The model under review builds one solid part; all positions refer to its coordinate system, in mm. Coordinates: 2 decimals unless noted, no trailing zeros. Write each loop counter-clockwise with the first axis right and the second up, starting at its lowest first coordinate (ties: lowest second). Pieces come first, ordered by that corner, then holes. Notation, with made-up numbers: M 76.5,-32 L 118.5,-32 A21 cw 118.5,-14 Z; hole C -36.5,-17 d3. An arc over 180 degrees is marked long. Answer as a JSON object with one key per item and string values.
Autodesk Inventor part; units mm, degrees
ref_plane "YZ Plane" through (0, 0, 0) normal (1, 0, 0) x (0, 1, 0)
ref_plane "XZ Plane" through (0, 0, 0) normal (0, 1, 0) x (-1, 0, 0)
ref_plane "XY Plane" through (0, 0, 0) normal (0, 0, 1) x (1, 0, 0)
sketch "Sketch1" plane through (0, 0, 0) normal (1, 0, 0) x (0, 1, 0)
  line L0 (0, 0) -> (107.95, 0)
  line L1 (107.95, 0) -> (107.95, -444.5)
  line L2 (107.95, -444.5) -> (0, -444.5)
  line L3 (0, -444.5) -> (0, 0)
  circle A0 centre (31.75, -50.8) radius 6.3627
  circle A1 centre (31.75, -393.7) radius 6.3627
  circle A2 centre (92.6338, -165.5318) radius 1.5875
  circle A3 centre (76.6318, -165.5318) radius 1.5875
  circle A4 centre (15.3162, -278.9682) radius 1.5875
  circle A5 centre (31.3182, -278.9682) radius 1.5875
  dimension "d0" = 107.95
  dimension "d1" = 444.5
  dimension "d2" = 12.7254
  dimension "d3" = 31.75
  dimension "d4" = 50.8
  dimension "d5" = 50.8
  dimension "d22" = 165.5318
  dimension "d23" = 3.175
  dimension "d24" = 15.3162
  dimension "d25" = 3.175
  dimension "d26" = 16.002
  dimension "d27" = 165.5318
  dimension "d28" = 3.175
  dimension "d29" = 15.3162
  dimension "d30" = 165.5318
  dimension "d31" = 3.175
  dimension "d32" = 16.002
  dimension "d33" = 165.5318
extrude "Extrusion1" add sketch "Sketch1" along normal blind 4.7625 contours L0 L1 L2 L3 | A2 | A3 | A4 | A5
chamfer "Chamfer1" distance 38.1 angle 45 1 edges at (2.3813, 0, 0)
chamfer "Chamfer2" distance 38.1 angle 45 1 edges at (2.3813, 0, -444.5)
sketch "Sketch2" plane through (4.7625, 0, 0) normal (1, 0, 0) x (0, 0, -1)
  line L0 (444.5, 38.1) -> (406.4, 0)
  line L1 (444.5, 38.1) -> (444.5, 107.95)
  line L2 (444.5, 107.95) -> (0, 107.95)
  line L3 (0, 107.95) -> (0, 38.1)
  line L4 (38.1, 0) -> (0, 38.1)
  line L5 (38.1, 0) -> (406.4, 0)
  circle A0 centre (393.7, 31.75) radius 6.3627
  circle A1 centre (50.8, 31.75) radius 6.3627
  circle A2 centre (120.65, 38.989) radius 6.3627
  circle A3 centre (323.85, 68.961) radius 6.3627
  point P0 (0, 0)
  dimension "d14" = 12.7254
  dimension "d15" = 120.65
  dimension "d17" = 12.7254
  dimension "d19" = 120.65
  dimension "d78" = 38.989
  dimension "d79" = 38.989
extrude "Extrusion2" cut sketch "Sketch2" against normal blind 25.4 contours A2 | A3
sketch "Sketch6" plane through (4.7625, 0, 0) normal (1, 0, 0) x (0, 0, -1)
  circle A0 centre (120.65, 38.989) radius 6.3627
  circle A1 centre (323.85, 68.961) radius 6.3627
  line L0 (444.5, 38.1) -> (406.4, 0)
  line L1 (444.5, 38.1) -> (444.5, 107.95)
  line L2 (444.5, 107.95) -> (0, 107.95)
  line L3 (0, 107.95) -> (0, 38.1)
  line L4 (38.1, 0) -> (0, 38.1)
  line L5 (38.1, 0) -> (406.4, 0)
  circle A2 centre (393.7, 31.75) radius 6.3627
  circle A3 centre (50.8, 31.75) radius 6.3627
  point P0 (0, 0)
  point P1 (165.7604, 16.002)
  point P2 (165.7604, 48.006)
  point P3 (278.7396, 91.948)
  point P4 (278.7396, 59.944)
  dimension "d80" = 45.1104
  dimension "d81" = 45.1104
  dimension "d82" = 32.004
  dimension "d83" = 16.002
  dimension "d84" = 32.004
  dimension "d85" = 16.002
  dimension "d86" = 45.1104
  dimension "d87" = 45.1104
hole "Hole1" at (4.7625, 16.002, -165.7604) at (4.7625, 48.006, -165.7604) at (4.7625, 91.948, -278.7396) at (4.7625, 59.944, -278.7396) direction (-1, 0, 0) diameter 3.81 end through all
sketch "Sketch7" plane through (4.7625, 0, 0) normal (1, 0, 0) x (0, 0, -1)
  circle A0 centre (278.7396, 91.948) radius 1.905
  circle A1 centre (165.7604, 16.002) radius 1.905
  circle A2 centre (165.7604, 48.006) radius 1.905
  circle A3 centre (278.7396, 59.944) radius 1.905
  circle A4 centre (120.65, 38.989) radius 6.3627
  circle A5 centre (323.85, 68.961) radius 6.3627
  line L0 (444.5, 38.1) -> (406.4, 0)
  line L1 (444.5, 38.1) -> (444.5, 107.95)
  line L2 (444.5, 107.95) -> (0, 107.95)
  line L3 (0, 107.95) -> (0, 38.1)
  line L4 (38.1, 0) -> (0, 38.1)
  line L5 (38.1, 0) -> (406.4, 0)
  circle A6 centre (393.7, 31.75) radius 6.3627
  circle A7 centre (50.8, 31.75) radius 6.3627
  line L6 (395.7601, 93.9533) -> (387.35, 98.425)
  circle A8 centre (387.35, 98.425) radius 9.525
  point P0 (0, 0)
  point P1 (80.9625, 92.075)
  point P2 (90.4875, 92.075)
  dimension "d102" = 19.05
  dimension "d95" = 15.875
  dimension "d96" = 15.875
  dimension "d97" = 9.525
  dimension "d98" = 80.9625
  dimension "d99" = 9.525
  dimension "d100" = 57.15
  dimension "d101" = 28
hole "Hole2" at (4.7625, 92.075, -80.9625) at (4.7625, 92.075, -90.4875) at (4.7625, 98.425, -387.35) at (4.7625, 93.9533, -395.7601) direction (-1, 0, 0) diameter 3.81 depth 25.4 tip angle 118
sketch "Sketch8" plane through (4.7625, 0, 0) normal (1, 0, 0) x (0, 0, -1)
  circle A0 centre (387.35, 98.425) radius 1.905
  circle A1 centre (80.9625, 92.075) radius 1.905
  circle A2 centre (90.4875, 92.075) radius 1.905
  circle A3 centre (395.7601, 93.9533) radius 1.905
  circle A4 centre (278.7396, 91.948) radius 1.905
  circle A5 centre (165.7604, 16.002) radius 1.905
  circle A6 centre (165.7604, 48.006) radius 1.905
  circle A7 centre (278.7396, 59.944) radius 1.905
  circle A8 centre (120.65, 38.989) radius 6.3627
  circle A9 centre (323.85, 68.961) radius 6.3627
  line L0 (444.5, 38.1) -> (406.4, 0)
  line L1 (444.5, 38.1) -> (444.5, 107.95)
  line L2 (444.5, 107.95) -> (0, 107.95)
  line L3 (0, 107.95) -> (0, 38.1)
  line L4 (38.1, 0) -> (0, 38.1)
  line L5 (38.1, 0) -> (406.4, 0)
  circle A10 centre (393.7, 31.75) radius 6.3627
  circle A11 centre (50.8, 31.75) radius 6.3627
  point P0 (0, 0)
  point P1 (101.6, 103.505)
  point P2 (342.9, 103.505)
  point P3 (127, 4.445)
  point P4 (317.5, 4.445)
  dimension "d110" = 4.445
  dimension "d111" = 4.445
  dimension "d112" = 101.6
  dimension "d113" = 101.6
  dimension "d114" = 4.445
  dimension "d115" = 4.445
  dimension "d123" = 127
  dimension "d124" = 127
hole "Hole3" at (4.7625, 103.505, -101.6) at (4.7625, 103.505, -342.9) at (4.7625, 4.445, -127) at (4.7625, 4.445, -317.5) direction (-1, 0, 0) diameter 3.81 depth 25.4 tip angle 118
equation "\"d19\" = d15"
properties part number "DriveTrain3.0"
(1) Draft analysis for pull direction Y (two halves, no side actions). For faces 1 (the face through (2.4, 19.3, -425.7)), 2 (the face through (0, 53, -219)), 3 (the face through (2.415, 66.524, -329.728)), state which applies: released by +Y, released by -Y, zero draft, split by the parting line, or undercut.
Results list:
{"face 1": "released by -Y", "face 2": "zero draft", "face 3": "undercut"}
(2) Add section A-A on z = -50.8. Give the boundary of the cut face in (x, y).
Results list:
{"outline": "M 0,0 L 4.76,0 L 4.76,25.39 L 0,25.39 Z; M 0,38.11 L 4.76,38.11 L 4.76,107.95 L 0,107.95 Z"}
(3) Add section B-B on x = 1.75. Count the separate pieces of the cut face and the enclosed holes in it, and give its area (3 significant figures).
Results list:
{"separate pieces": "1", "enclosed holes": "16", "area": "45,900 mm²"}
(4) Wall thickness on line 1 along Z through (x, y) = (3.3, 69.5); line 2 along Y through (x, z) = (3.15, -277.5); line 3 along Y through (x, z) = (3.15, -323.85): over which ranges is each line inside the solid? List them lowest first. Write a range as from..to.
Results list:
{"line 1": "-444.5..-330.19, -317.51..0", "line 2": "0..58.5, 61.39..90.5, 93.39..107.95", "line 3": "0..62.6, 75.32..107.95"}
(5) For pin 1 Ø2.5 at (y, z) = (103.505, -342.9) entering from +X, flat-tipped, find the tip position at first contact; note if it passes through.
Results list:
{"pin 1": "through"}
